Autodesk Fusion 360 part; units mm, degrees
sketch "Arm triangle" plane through (0, 0, 0) normal (0, 1, 0) x (1, 0, 0)
  line L0 (0, 0) -> (0, -76)
  line L1 (0, -76) -> (115, -76)
  line L2 (115, -76) -> (0, 0)
extrude "Arm triangle (1)" add sketch "Arm triangle" along normal mid plane 40
sketch "Hook plate" plane through (0, 0, 0) normal (0, 1, 0) x (1, 0, 0)
  line L0 (0, 0) -> (6, 0)
  line L1 (6, 0) -> (6, -76)
  line L2 (6, -76) -> (0, -76)
  line L3 (0, -76) -> (0, 0)
extrude "Hook plate (1)" add sketch "Hook plate" along normal mid plane 40
sketch "Saddle boss" plane through (0, 0, 0) normal (0, 1, 0) x (1, 0, 0)
  circle A0 centre (115, -76) radius 22.7
extrude "Saddle boss (1)" add sketch "Saddle boss" along normal mid plane 40
sketch "Lightening cutout" plane through (0, 0, 0) normal (0, 1, 0) x (1, 0, 0)
  line L0 (14, -26.0332) -> (14, -62)
  line L1 (14, -62) -> (68.4235, -62)
  line L2 (68.4235, -62) -> (14, -26.0332)
extrude "Lightening cutout (1)" cut sketch "Lightening cutout" along normal mid plane 50
sketch "Rod pocket" plane through (0, 0, 0) normal (0, 1, 0) x (1, 0, 0)
  circle A0 centre (115, -76) radius 17.1
extrude "Rod pocket (1)" cut sketch "Rod pocket" along normal mid plane 50
sketch "Rod drop-in opening" plane through (0, 0, 0) normal (0, 1, 0) x (1, 0, 0)
  line L0 (97.9, -76) -> (132.1, -76)
  line L1 (132.1, -76) -> (132.1, -103.7)
  line L2 (132.1, -103.7) -> (97.9, -103.7)
  line L3 (97.9, -103.7) -> (97.9, -76)
extrude "Rod drop-in opening (1)" cut sketch "Rod drop-in opening" along normal mid plane 50
sketch "Hook profiles" plane through (0, 0, 0) normal (0, 1, 0) x (1, 0, 0)
  line L0 (0, -74) -> (-6.8, -74)
  line L1 (-6.8, -74) -> (-6.8, -57)
  line L2 (-6.8, -57) -> (-2.8, -57)
  line L3 (-2.8, -57) -> (-2.8, -69)
  line L4 (-2.8, -69) -> (0, -69)
  line L5 (0, -69) -> (0, -74)
  line L6 (0, -48.6) -> (-6.8, -48.6)
  line L7 (-6.8, -48.6) -> (-6.8, -31.6)
  line L8 (-6.8, -31.6) -> (-2.8, -31.6)
  line L9 (-2.8, -31.6) -> (-2.8, -43.6)
  line L10 (-2.8, -43.6) -> (0, -43.6)
  line L11 (0, -43.6) -> (0, -48.6)
  line L12 (0, -23.2) -> (-6.8, -23.2)
  line L13 (-6.8, -23.2) -> (-6.8, -6.2)
  line L14 (-6.8, -6.2) -> (-2.8, -6.2)
  line L15 (-2.8, -6.2) -> (-2.8, -18.2)
  line L16 (-2.8, -18.2) -> (0, -18.2)
  line L17 (0, -18.2) -> (0, -23.2)
extrude "Hook slab" add sketch "Hook profiles" along normal mid plane 27.8
extrude "Hook column split" cut sketch "Hook profiles" along normal mid plane 23
Geometry: final body of the model. Coordinates: model frame, mm. A direction names the side the tool comes from. Coordinates: 2 decimals unless noted, no trailing zeros. Write each loop counter-clockwise with the first axis right and the second up, starting at its lowest first coordinate (ties: lowest second). Pieces come first, ordered by that corner, then holes. Notation, with made-up numbers: M 87,61 L 100,61 A24 cw 100,73 Z; hole C 57,20 d5. An arc over 180 degrees is marked long. Use CSV: the item, a comma, the result in double quotes. Start each with the question number.
1. First-contact query: P1, Ø1, axis at x = 82, y = -3, coming from the +Z side; P2, Ø12, axis at y = 10, z = 35, coming from the -X side; P3, Ø4, axis at x = 105, y = 3, coming from the -Z side; P4, Ø1.2, axis at x = -2.5, y = -12.5, coming from the +Z side. Flat tips, straight axial feed; report the tip coordinate or a pass-through.
2. Cut plane B-B on z = 29. Return the cut outline in (x, y).
3. Reachability of faces 4 (the face through (-4, -11.5, 16)), 5 (the face through (97.9, 0, 84)), 6 (the face through (41, 0, 62)) from +Z, -Z, +X, -X, +Y, -Y: full face, straight path, thin tool, end or side. Return the list, or none.
4. Cut plane A-A on y = 17.5. Return the cut outline in (x, z), plus the area to 3 significant figures.
5. Cut plane C-C on x = 115. Return the cut outline in (y, z).
6. Mould query, pull axis Z, two halves, no side actions, for faces 1 (the face through (115.376, 0.28, 58.904)), 2 (the face through (41.593, -0.28, 44.268)), 3 (the face through (51.66, -0.28, 34.14)). Classes: pulls with the +Z half, pulls with the -Z half, needs draft (parallel to the pull), parting line crosses it, or undercut.
7. Ray query, probe 1 along X at (y, z) = (7.5, 66); probe 2 along X at (y, z) = (10.5, 53); probe 3 along Z at (x, y) = (51, -2). Return the intervals inside material, ascending.
Entries:
1,P1,"z = 76"
1,P2,"x = -6.8"
1,P3,"z = 54.76"
1,P4,"z = 74"
2,outline,"M 0,-20 L 14,-20 L 14,20 L 0,20 Z; M 18.49,-20 L 43.88,-20 L 43.88,20 L 18.49,20 Z"
3,face 4,"+Z, -Z, -X"
3,face 5,"+Z, +Y, -Y"
3,face 6,"+Y, -Y"
4,outline,"M 0,0 L 6,0 L 6,3.97 L 96.06,63.48 A22.7 ccw long 132.1,90.93 L 132.1,76 A17.1 cw 97.9,76 L 97.9,90.93 A22.7 ccw 92.3,76 L 0,76 Z; hole M 14,26.03 L 68.42,62 L 14,62 Z"
4,area,"3,720 mm²"
5,outline,"M -20,53.3 L 20,53.3 L 20,58.9 L -20,58.9 Z"
6,face 1,"pulls with the +Z half"
6,face 2,"undercut"
6,face 3,"pulls with the -Z half"
7,probe 1,"0 to 101.13, 128.87 to 135.38"
7,probe 2,"0 to 14, 54.81 to 80.2"
7,probe 3,"33.7 to 50.49, 62 to 76"
